Source: CAD feature listing. Evaluate the final solid. Frame: model axes, mm. Face numbers are marked on the shaded views. A direction names the side the tool comes from. Coordinates: 2 decimals unless noted, no trailing zeros. Loops run counter-clockwise (first coordinate to the right, second up) from the corner with the lowest first, then second, coordinate; pieces in that order, holes last.
Item 1: Pin query (flat end, axial travel): pin 1 Ø9.5 at (x, z) = (45, 0) entering from -Y; pin 2 Ø9.5 at (x, z) = (44.5, 4) entering from -Y; pin 3 Ø0.8 at (x, z) = (31.5, -1) entering from +Y; pin 4 Ø0.6 at (x, z) = (-12, -27.5) entering from -Y. Return the tip coordinate at first contact, or that it passes through.
Item 2: Section query D-D, the plane y = 35. Return the cut outline in (x, z), then the cut area to 3 significant figures.
Item 3: Reachability of the marked faces 1, 2, 3 and 4 from +Z, -Z, +X, -X, +Y, -Y: full face, straight path, thin tool, end or side. Return the list, or none.
Item 4: Line query: probe 1 along Y at (x, z) = (-15, -36); probe 2 along Y at (x, z) = (0, -14); probe 3 along X at (y, z) = (13, -41). Output: solid intervals per line, ascending.
Item 5: Section query A-A, the plane z = -21. Return the cut outline in (x, y), then the cut area to 3 significant figures.
Item 6: Section query B-B, the plane x = 0. Return the cut outline in (y, z), then the cut area to 3 significant figures.
Item 7: Section query C-C, the plane z = 17. Return the cut outline in (x, y), then the cut area to 3 significant figures.
Item 8: Pull-direction query (X, two-part tool) for the marked faces 5, 6, 7 and 8; classes: +X half, -X half, draft (parallel to the pull), parting line (faces both ways), or undercut.
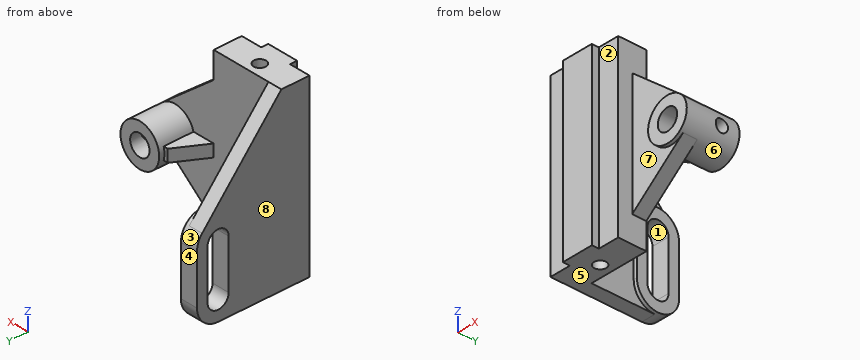
```python
from build123d import *

# Parameters (mm, degrees)
SKETCH_1_R           = 3.5
EXTRUDE_1_DEPTH      = 50
EXTRUDE_2_DEPTH      = 8
EXTRUDE_3_DEPTH      = 10
EXTRUDE_4_DEPTH      = 8
EXTRUDE_5_DEPTH      = 20
EXTRUDE_5_DEPTH_BACK = 10
SKETCH_3_3_R         = 12
SKETCH_3_3_R_2       = 6
RIB_START            = -3.5
RIB_12_DEPTH         = 7
CUT_EXTRUDE_START    = 49.873397053
CUT_EXTRUDE_1_DEPTH  = 7.126602664


# Read off the part's stored shape, not the designer's step: 筋12, 切除-拉伸1
with BuildPart() as part:
    # 草图1 → 凸台-拉伸1 (new, symmetric)
    with BuildSketch(Plane.XY):
        Polygon((21, 7), (-21, 7), (-21, -9), (-9, -9), (-9, -13), (9, -13), (9, -9), (21, -9), align=None)
        Circle(SKETCH_1_R, mode=Mode.SUBTRACT)
    extrude(amount=EXTRUDE_1_DEPTH, both=True)

    # 草图2 → 凸台-拉伸2 (add)
    with BuildSketch(Plane.ZY.offset(21)):
        with BuildLine():
            Line((-50, 43), (-50, 7))
            Line((-50, 7), (50, 7))
            Line((50, 7), (-2.152816021, 52.078639964))
            ThreePointArc((-2.152816021, 52.078639964), (1.245969935, 38.813335431), (-10, 31))
            Line((-10, 31), (-38, 31))
            ThreePointArc((-38, 31), (-46.485281374, 34.514718626), (-50, 43))
        make_face()
    extrude(amount=-EXTRUDE_2_DEPTH)

    # 草图2<3> → 凸台-拉伸3 (add)
    with BuildSketch(Plane.ZY.offset(21)):
        with BuildLine():
            Line((-10, 55), (-38, 55))
            ThreePointArc((-38, 55), (-50, 43), (-38, 31))
            Line((-38, 31), (-10, 31))
            ThreePointArc((-10, 31), (2, 43), (-10, 55))
        make_face()
        with BuildLine():
            ThreePointArc((-38, 49), (-44, 43), (-38, 37))
            Line((-38, 37), (-10, 37))
            ThreePointArc((-10, 37), (-4, 43), (-10, 49))
            Line((-10, 49), (-38, 49))
        make_face(mode=Mode.SUBTRACT)
    extrude(amount=-EXTRUDE_3_DEPTH)

    # 草图3 → 凸台-拉伸4 (add)
    with BuildSketch(Plane(origin=(0, 7, 0), x_dir=(1, 0, 0), z_dir=(0, 1, 0))):
        with BuildLine():
            Line((33, 0), (21, 0))
            Line((21, 0), (21, -35))
            Line((21, -35), (52.573920737, -9.307831362))
            ThreePointArc((52.573920737, -9.307831362), (39.846702456, -10.837136357), (33, 0))
        make_face()
        with BuildLine():
            Line((21, 35), (21, 0))
            Line((21, 0), (33, 0))
            ThreePointArc((33, 0), (39.846702456, 10.837136357), (52.573920737, 9.307831362))
            Line((52.573920737, 9.307831362), (21, 35))
        make_face()
    extrude(amount=-EXTRUDE_4_DEPTH)

    # 草图3<3> → 凸台-拉伸5 (add, two sides: drawn at the far end of the back side and taken through both)
    with BuildSketch(Plane(origin=(0, 7, 0), x_dir=(1, 0, 0), z_dir=(0, 1, 0)).offset(-EXTRUDE_5_DEPTH_BACK)):
        with Locations(Location((45, 0, 0), (0, 0, 270))):
            Circle(SKETCH_3_3_R)
        with Locations(Location((45, 0, 0), (0, 0, 270))):
            Circle(SKETCH_3_3_R_2, mode=Mode.SUBTRACT)
    extrude(amount=EXTRUDE_5_DEPTH + EXTRUDE_5_DEPTH_BACK)

    # 筋12 outline → 筋12 (add)
    with BuildSketch(Plane.XY.offset(RIB_START)):
        Polygon((35, 24), (31, 24), (21, 7), (35, 7), align=None)
    extrude(amount=RIB_12_DEPTH)

    # 切除-拉伸1 outline → 切除-拉伸1 (cut)
    with BuildSketch(Plane(origin=(0, 0, 0), x_dir=(0, 0, -1), z_dir=(1, 0, 0)).offset(CUT_EXTRUDE_START)):
        with BuildLine():
            add(Edge.make_bspline(
                [(-3.5, 17), (-3.5, 17.930374798), (-3.116526668, 18.833354303), (-1.832705903, 20.11690801), (-0.921038324, 20.499404533), (0.916507131, 20.500594001), (1.828824497, 20.121110709), (3.121641798, 18.827917827), (3.499603295, 17.918268751), (3.500396051, 16.084757844), (3.121933694, 15.173019649), (1.831002297, 13.880423461), (0.924027469, 13.500295231), (-0.921789584, 13.499705127), (-1.831835104, 13.88257801), (-3.116022585, 15.165785464), (-3.5, 16.069625202), (-3.5, 17)],
                knots=[0, 0, 0, 0, 0.125, 0.125, 0.25, 0.25, 0.375, 0.375, 0.5, 0.5, 0.625, 0.625, 0.75, 0.75, 0.875, 0.875, 1, 1, 1, 1], degree=3))
        make_face()
    extrude(amount=CUT_EXTRUDE_1_DEPTH, mode=Mode.SUBTRACT)


solid = part.part
```
Verdict:
1. pin 1: passes through
1. pin 2: stops at y = -3
1. pin 3: stops at y = 24
1. pin 4: stops at y = -9
2. outline: (-21, -50) - (-13, -50) - (-13, -46.94) - (-11, -46.94) - (-11, -1.06) - (-13, -1.06) - (-13, 17.61) - (-21, 17.61) - close
2. area: 633 mm2
3. face 1: +X, -X
3. face 2: +Z, -Z, +X, -Y
3. face 3: +Z, +X
3. face 4: +Z, -Z, +X, -X, +Y
4. probe 1: y = -9 to 37, 49 to 55
4. probe 2: y = -13 to -3.5, 3.5 to 7
4. probe 3: x = -21 to -13
5. outline: (-21, -9) - (-9, -9) - (-9, -13) - (9, -13) - (9, -9) - (21, -9) - (21, -1) - (38.21, -1) - (38.21, 7) - (-13, 7) - (-13, 31) - (-11, 31) - (-11, 37) - (-21, 37) - close; (-21, 49) - (-11, 49) - (-11, 55) - (-21, 55) - close; hole circle Ø7 at (0, 0)
5. area: 1,160 mm2
6. outline: (-13, -50) - (-3.5, -50) - (-3.5, 50) - (-13, 50) - close; (3.5, -50) - (7, -50) - (7, 50) - (3.5, 50) - close
6. area: 1,300 mm2
7. outline: (-21, -9) - (-9, -9) - (-9, -13) - (9, -13) - (9, -9) - (21, -9) - (21, -1) - (43.12, -1) - (43.12, 7) - (-13, 7) - (-13, 35.52) - (-21, 35.52) - close; hole circle Ø7 at (0, 0)
7. area: 1,110 mm2
8. face 5: draft
8. face 6: undercut
8. face 7: undercut
8. face 8: -X half
